Work out the finished part from the listing and answer in its coordinate system (mm). Face numbers are marked on the shaded views. A direction names the side the tool comes from. Round coordinates to 2 decimals unless told otherwise and drop trailing zeros. Order: outer loops, then holes, each group sorted by start corner. A loop starts at its lowest first (then second) coordinate and runs counter-clockwise, first axis right, second up. Notation, with made-up numbers: M 51.5,8.5 L 63.5,8.5 A22 ccw 63.5,17.5 Z; hole C 50.25,67.25 d2. An arc over 180 degrees is marked long. Return JSON: item names as keys, results as strings.
from build123d import *

# Parameters (mm, degrees)
SKETCH1_W           = 41
SKETCH1_H           = 21
BOSS_EXTRUDE1_DEPTH = 25
BOSS_EXTRUDE2_DEPTH = 3
SKETCH5_W           = 41
SKETCH5_H           = 21
BOSS_EXTRUDE3_DEPTH = 9
SKETCH6_R           = 2
CUT_EXTRUDE1_DEPTH  = 9
SKETCH7_R           = 2
CUT_EXTRUDE2_DEPTH  = 9
SKETCH8_R           = 10.5
BOSS_EXTRUDE4_DEPTH = 8


with BuildPart() as part:
    # Sketch1 → Boss-Extrude1 (new body)
    with BuildSketch(Plane.XY):
        with Locations((-25.101821211, -5.243485894)):
            Rectangle(SKETCH1_W, SKETCH1_H)
    extrude(amount=BOSS_EXTRUDE1_DEPTH)

    # Sketch4 → Boss-Extrude2 (add)
    with BuildSketch(Plane.XY.offset(25)):
        Polygon((-4.601821211, 5.256514106), (-45.601821211, 5.256514106), (-53.601821211, 5.256514106), (-53.601821211, -15.743485894), (-45.601821211, -15.743485894), (-4.601821211, -15.743485894), (3.398178789, -15.743485894), (3.398178789, 5.256514106), align=None)
    extrude(amount=BOSS_EXTRUDE2_DEPTH)

    # Sketch5 → Boss-Extrude3 (add)
    with BuildSketch(Plane.XY.offset(28)):
        with Locations((-25.101821211, -5.243485894)):
            Rectangle(SKETCH5_W, SKETCH5_H)
    extrude(amount=BOSS_EXTRUDE3_DEPTH)

    # Sketch6 → Cut-Extrude1 (cut)
    with BuildSketch(Plane.XY.offset(28)):
        with Locations((-50.601821211, -10.743485894)):
            Circle(SKETCH6_R)
        with Locations((-50.601821211, 0.256514106)):
            Circle(SKETCH6_R)
    extrude(amount=-CUT_EXTRUDE1_DEPTH, mode=Mode.SUBTRACT)

    # Sketch7 → Cut-Extrude2 (cut)
    with BuildSketch(Plane.XY.offset(28)):
        with Locations((0.398178789, -10.743485894)):
            Circle(SKETCH7_R)
        with Locations((0.398178789, 0.256514106)):
            Circle(SKETCH7_R)
    extrude(amount=-CUT_EXTRUDE2_DEPTH, mode=Mode.SUBTRACT)

    # Sketch8 → Boss-Extrude4 (add)
    with BuildSketch(Plane.XY.offset(37)):
        with Locations(Location((-15.601821211, -5.243485894, 0), (0, 0, 270))):
            Circle(SKETCH8_R)
    extrude(amount=BOSS_EXTRUDE4_DEPTH)


solid = part.part
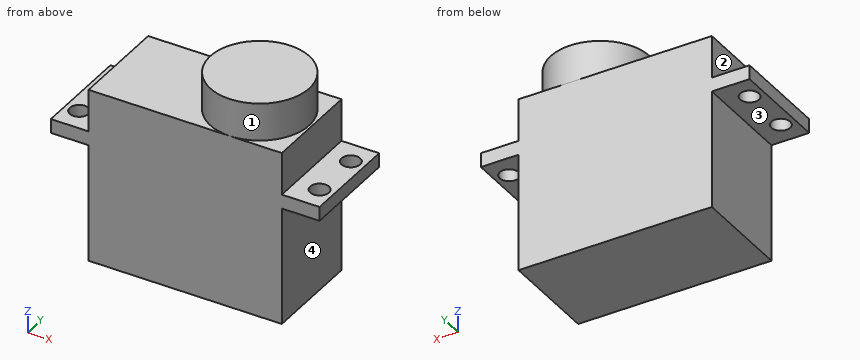
Item 1: Find section D-D (y = -5). Determine the outline of the cut face in (x, z).
Output:
{"outline": "M -53.6,25 L -45.6,25 L -45.6,0 L -4.6,0 L -4.6,25 L 3.4,25 L 3.4,28 L -4.6,28 L -4.6,37 L -5.1,37 L -5.1,45 L -26.1,45 L -26.1,37 L -45.6,37 L -45.6,28 L -53.6,28 Z"}
Item 2: Find section B-B (x = -25). Determine the outline of the cut face in (y, z).
Output:
{"outline": "M -15.74,0 L 5.26,0 L 5.26,37 L -0.56,37 L -0.56,45 L -9.93,45 L -9.93,37 L -15.74,37 Z"}
Item 3: Each of these flat-tipped pins is pushed along its axis until it touches: pin 1 (2.5 mm diameter, centred on x = 0, y = -3.5, fed in from +Z); pin 2 (9 mm diameter, centred on x = -48.5, y = -2.5, fed in from +Z); pin 3 (6.5 mm diameter, centred on x = -50.6, y = -10.74, fed in from -Z); pin 4 (3.5 mm diameter, centred on x = 0.4, y = 0.26, fed in from -Z). Where does it stop, or does it pass through?
Output:
{"pin 1": "stops at z = 28", "pin 2": "stops at z = 37", "pin 3": "stops at z = 25", "pin 4": "passes through"}
Item 4: Find section A-A (y = -11.5). Determine the outline of the cut face in (x, z), plus the area to 3 significant figures.
Output:
{"outline": "M -53.6,25 L -52.45,25 L -52.45,28 L -53.6,28 Z; M -48.75,25 L -45.6,25 L -45.6,0 L -4.6,0 L -4.6,25 L -1.45,25 L -1.45,28 L -4.6,28 L -4.6,37 L -7.17,37 L -7.17,45 L -24.03,45 L -24.03,37 L -45.6,37 L -45.6,28 L -48.75,28 Z; M 2.25,25 L 3.4,25 L 3.4,28 L 2.25,28 Z", "area": "1,680 mm^2"}
Item 5: Consider line 1 along X through (y, z) = (-2.25, 18.5); line 2 along Z through (x, y) = (-26.5, -9.5); line 3 along X through (y, z) = (-5, 41). Determine where each line is inside the solid, lowest interval first. Write a range as [from, to].
Output:
{"line 1": "x = [-45.6, -4.6]", "line 2": "z = [0, 37]", "line 3": "x = [-26.1, -5.1]"}
Item 6: Find section C-C (z = 29.5). Determine the outline of the cut face in (x, y), plus the area to 3 significant figures.
Output:
{"outline": "M -45.6,-15.74 L -4.6,-15.74 L -4.6,5.26 L -45.6,5.26 Z", "area": "861 mm^2"}
Item 7: Which of the six approach directions +Z, -Z, +X, -X, +Y, -Y give full straight-line access (tool end or side, diameter ignored) to the marked faces 1, 2, 3 and 4?
Output:
{"face 1": "+Z", "face 2": "+Z, -X, +Y, -Y", "face 3": "-Z, -X, +Y, -Y", "face 4": "-Z, +X, +Y, -Y"}
